from build123d import *

# Parameters (mm, degrees)
CLONE2D014_W    = 772
CLONE2D014_H    = 208
PAD015_DEPTH    = 19
SKETCH039_W     = 622
SKETCH039_H     = 108
POCKET015_DEPTH = 10


with BuildPart() as part:
    # Clone2D014 → Pad015 (new body)
    with BuildSketch(Plane.XZ):
        with Locations((386, 104)):
            Rectangle(CLONE2D014_W, CLONE2D014_H)
    extrude(amount=PAD015_DEPTH)

    # Sketch039 (on Face6 of Pad015) → Pocket015 (cut)
    with BuildSketch(Plane.XZ.offset(19)):
        with Locations((386, 104)):
            Rectangle(SKETCH039_W, SKETCH039_H)
    extrude(amount=-POCKET015_DEPTH, mode=Mode.SUBTRACT)

    # Clone2D015 → Revolution008 (revolve)
    with BuildSketch(Plane(origin=(175, -9, 104), x_dir=(1, 0, 0), z_dir=(0, 0, 1))):
        with BuildLine():
            Line((0, 0), (0, -20))
            add(Edge.make_bspline(
                [(0, -20), (-18, -20), (-18, -9.133286), (-4.506424, -9.133286), (-7.5, 0)],
                knots=[0, 0, 0, 0, 0.5, 1, 1, 1, 1], degree=3, weights=[7, 6.116989, 5.810816, 6.060123, 5.999522]))
            Line((-7.5, 0), (0, 0))
        make_face()
    revolve(axis=Axis((175, -9, 104), (0, 1, 0)))

    # Clone2D016 → Revolution009 (revolve)
    with BuildSketch(Plane(origin=(574, -9, 104), x_dir=(1, 0, 0), z_dir=(0, 0, 1))):
        with BuildLine():
            Line((0, 0), (0, -20))
            add(Edge.make_bspline(
                [(0, -20), (-18, -20), (-18, -9.133286), (-4.506424, -9.133286), (-7.5, 0)],
                knots=[0, 0, 0, 0, 0.5, 1, 1, 1, 1], degree=3, weights=[7, 6.116989, 5.810816, 6.060123, 5.999522]))
            Line((-7.5, 0), (0, 0))
        make_face()
    revolve(axis=Axis((574, -9, 104), (0, 1, 0)))


with BuildPart() as part_1:
    # Body019 placement: moved
    add(part.part.moved(Location((394, 0, 236))))


solid = part_1.part
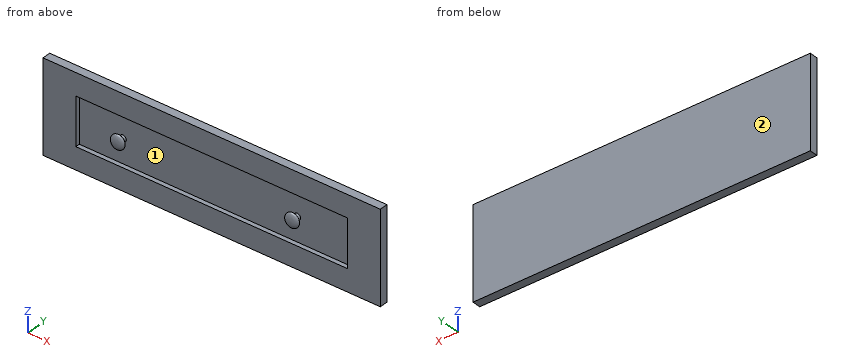
The listing builds one solid part. Answer for the finished solid, in the listing's coordinates (mm). Face numbers are marked on the shaded views. Coordinates: 2 decimals unless noted, no trailing zeros. Loops run counter-clockwise (first coordinate to the right, second up) from the corner with the lowest first, then second, coordinate; pieces in that order, holes last. Notation, with made-up numbers: M 13,31.5 L 62,31.5 A27 cw 62,65.5 Z; hole C -26,48.25 d7. An arc over 180 degrees is marked long. Answer in a Markdown table with one row per item.
1) Find section C-C (z = 265). Determine the outline of the cut face in (x, y), then the cut area to 3 significant figures.
Answers below:
| item | result |
|---|---|
| outline | M 394,-19 L 1166,-19 L 1166,0 L 394,0 Z |
| area | 14,700 mm^2 |
2) Find section B-B (x = 912.5). Determine the outline of the cut face in (y, z), then the cut area to 3 significant figures.
Answers below:
| item | result |
|---|---|
| outline | M -19,236 L 0,236 L 0,444 L -19,444 L -19,394 L -9,394 L -9,286 L -19,286 Z |
| area | 2,870 mm^2 |
3) Determine the mould class of the marked faces 1 and 2 for opening direction X: released by +X, released by -X, zero draft, split by the parting line, or undercut.
Answers below:
| item | result |
|---|---|
| face 1 | undercut |
| face 2 | zero draft |
4) Find the intervals of material crossed by probe 1 along X at (y, z) = (-11.5, 301.5); probe 2 along Z at (x, y) = (895, -13.75); probe 3 along Y at (x, z) = (1105, 270), in increasing order.
Answers below:
| item | result |
|---|---|
| probe 1 | 394 to 469, 1091 to 1166 |
| probe 2 | 236 to 286, 394 to 444 |
| probe 3 | -19 to 0 |
5) Find section A-A (z = 315). Determine the outline of the cut face in (x, y), then the cut area to 3 significant figures.
Answers below:
| item | result |
|---|---|
| outline | M 394,-19 L 469,-19 L 469,-9 L 1091,-9 L 1091,-19 L 1166,-19 L 1166,0 L 394,0 Z |
| area | 8,450 mm^2 |
6) Given pin 1 (2 mm diameter, centred on x = 662, z = 375.5, fed in from -Y), flat-ended and moving along its own axis, determine where the tip first touches the part or whether it passes through.
Answers below:
| item | result |
|---|---|
| pin 1 | y = -9 |
